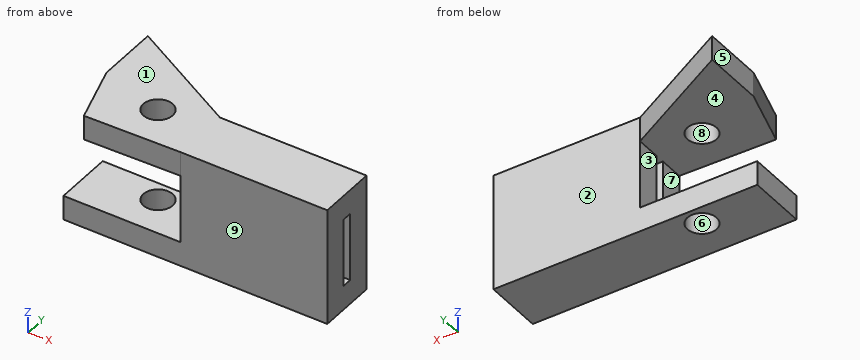
```python
from build123d import *

# Parameters (mm, degrees)
F0_W     = 7.62
F0_H     = 15.24
F1_DEPTH = 19.05
F2_T     = -3.175
F4_DEPTH = 3.175
F5_W     = 15.24
F5_H     = 7.62
F6_DEPTH = 3.175
F7_R     = 1.905
F8_DEPTH = 15.241


with BuildPart() as f1:
    # F0 (on Right) → F1 (new body)
    with BuildSketch(Plane.YZ):
        with Locations((-3.81, 7.62)):
            Rectangle(F0_W, F0_H)
    extrude(amount=F1_DEPTH)

    # F2
    f2_openings = [f1.faces().sort_by_distance(p)[0] for p in [
        (0, -3.81, 7.62),
        (19.05, -3.81, 7.62),
    ]]
    offset(amount=F2_T, openings=f2_openings)

    # F3 (on face) → F4 (join, through all)
    with BuildSketch(Plane.XY.offset(15.24)):
        Polygon((-12.3918876052, -7.9068467021), (0, -7.62), (0, 0), (-14.744957909, 8.033762686), (-14.744957909, 0), align=None)
    extrude(amount=-F4_DEPTH)

    # F5 (on face) → F6 (join, through all)
    with BuildSketch(Plane(origin=(0, 0, 0), x_dir=(1, 0, 0), z_dir=(0, 0, -1))):
        with Locations((-7.62, 3.81)):
            Rectangle(F5_W, F5_H)
    extrude(amount=-F6_DEPTH)

    # F7 (on face) → F8 (cut, through all)
    with BuildSketch(Plane.XY.offset(15.24)):
        with Locations((-6.35, -2.54)):
            Circle(F7_R)
    extrude(amount=-F8_DEPTH, mode=Mode.SUBTRACT)


solid = f1.part
```
Work out the finished part from the listing and answer in its coordinate system (mm). Face numbers are marked on the shaded views. A direction names the side the tool comes from. Give positions to 0.01 mm unless a question says otherwise; leave off trailing zeros. Loops run counter-clockwise (first coordinate to the right, second up) from the corner with the lowest first, then second, coordinate; pieces in that order, holes last. Notation, with made-up numbers: (-25, 12.25) -> (-3, 12.25) arc R27 ccw to (-3, 40.25) -> close; hole circle Ø10 at (33.25, -1.75). An arc over 180 degrees is marked (long way). One line per question, with ' | ' between items. Start each with the question number.
1) Determine the mould class of the marked faces 6, 7, 8 and 9 for opening direction Y: +Y half, -Y half, draft (parallel to the pull), parting line (faces both ways), or undercut.
2) Section C-C, the plane z = 9.25 is taken. Determine the outline of the cut face in (x, y) (3 decimals), then the cut area to 3 significant figures.
3) Section B-B, the plane z = 13.5 is taken. Determine the outline of the cut face in (x, y) (3 decimals), then the cut area to 3 significant figures.
4) Section D-D, the plane y = -2.54 is taken. Determine the outline of the cut face in (x, z) (3 decimals), then the cut area to 3 significant figures.
5) Each of these flat-tipped pins is pushed along its axis until it touches: pin 1 (3.5 mm diameter, centred on y = -1, z = 8.5, fed in from -X); pin 2 (4 mm diameter, centred on x = -6.5, z = 7, fed in from +Y); pin 3 (1 mm diameter, centred on y = 3.5, z = 13.5, fed in from -X); pin 4 (7 mm diameter, centred on x = 10, z = 7, fed in from +Y). Where does it stop, or does it pass through?
6) Section A-A, the plane x = 4.5 is taken. Determine the outline of the cut face in (y, z) (3 decimals).
7) Straight lines are drawn through the part: L1, parallel to Y at x = -6.35, z = 1.7 (3 decimals); L2, parallel to Z at x = -4.5, y = -4 (3 decimals); L3, parallel to Y at x = 4.5, z = 9.5 (3 decimals). For each, find the intervals that lie inside material, in ascending order.
8) For the marked faces 1, 2, 3, 4 and 5, determine the directions among +Z, -Z, +X, -X, +Y, -Y from which every point of the face is accessible in a straight line to the end or side of a thin tool.
Resolved:
1) face 6: undercut | face 7: draft | face 8: undercut | face 9: -Y half
2) outline: (0, -7.62) -> (19.05, -7.62) -> (19.05, -4.445) -> (0, -4.445) -> close; (0, -3.175) -> (19.05, -3.175) -> (19.05, 0) -> (0, 0) -> close | area: 121 mm2
3) outline: (-14.745, 0) -> (-12.392, -7.907) -> (0, -7.62) -> (19.05, -7.62) -> (19.05, 0) -> (0, 0) -> (-14.745, 8.034) -> close; hole circle Ø3.81 at (-6.35, -2.54) | area: 298 mm2
4) outline: (-15.24, 0) -> (-8.255, 0) -> (-8.255, 3.175) -> (-15.24, 3.175) -> close; (-13.989, 12.065) -> (-8.255, 12.065) -> (-8.255, 15.24) -> (-13.989, 15.24) -> close; (-4.445, 0) -> (19.05, 0) -> (19.05, 15.24) -> (-4.445, 15.24) -> (-4.445, 12.065) -> (0, 12.065) -> (0, 3.175) -> (-4.445, 3.175) -> close | area: 359 mm2
5) pin 1: x = 0 | pin 2: through | pin 3: x = -14.74 | pin 4: y = 0
6) outline: (-7.62, 0) -> (0, 0) -> (0, 15.24) -> (-7.62, 15.24) -> close; hole (-4.445, 3.175) -> (-3.175, 3.175) -> (-3.175, 12.065) -> (-4.445, 12.065) -> close
7) L1: -7.62 to -4.445, -0.635 to 0 | L2: 0 to 3.175, 12.065 to 15.24 | L3: -7.62 to -4.445, -3.175 to 0
8) face 1: +Z, +X, -X, +Y, -Y | face 2: -Z, +X, +Y | face 3: -X, +Y, -Y | face 4: -X | face 5: +Z, -Z, -X, +Y, -Y
